```python
from build123d import *

# Parameters (mm, degrees)
F0_R     = 5.25
F1_DEPTH = 12
F2_DEPTH = 11
F3_DEPTH = 12
F4_SIZE  = 1
F5_SIZE  = 1


with BuildPart() as f1:
    # F0 (on Top) → F1 (new body)
    with BuildSketch(Plane.XY):
        with BuildLine():
            ThreePointArc((4, -17.036725), (13.715867, -10.868533), (17.5, 0))
            ThreePointArc((17.5, 0), (-10.868533, 13.715867), (-4, -17.036725))
            ThreePointArc((-4, -17.036725), (0, -17.5), (4, -17.036725))
        make_face()
        Circle(F0_R, mode=Mode.SUBTRACT)
        Circle(F0_R)
        with BuildLine():
            ThreePointArc((2.727178, 1.25), (2.931001, 0.639713), (3, 0))
            ThreePointArc((3, 0), (-0.639713, -2.931001), (-2.727178, 1.25))
            ThreePointArc((-2.727178, 1.25), (0, 3), (2.727178, 1.25))
        make_face(mode=Mode.SUBTRACT)
        with BuildLine():
            ThreePointArc((-2.727178, 1.25), (-0.639713, -2.931001), (3, 0))
            ThreePointArc((3, 0), (2.931001, 0.639713), (2.727178, 1.25))
            Line((2.727178, 1.25), (-2.727178, 1.25))
        make_face()
        with BuildLine():
            Line((-2.727178, 1.25), (2.727178, 1.25))
            ThreePointArc((2.727178, 1.25), (0, 3), (-2.727178, 1.25))
        make_face()
    extrude(amount=F1_DEPTH)

    # F0 (on Top) → F2 (join)
    with BuildSketch(Plane.XY):
        Circle(F0_R)
        with BuildLine():
            ThreePointArc((2.727178, 1.25), (2.931001, 0.639713), (3, 0))
            ThreePointArc((3, 0), (-0.639713, -2.931001), (-2.727178, 1.25))
            ThreePointArc((-2.727178, 1.25), (0, 3), (2.727178, 1.25))
        make_face(mode=Mode.SUBTRACT)
        with BuildLine():
            Line((-2.727178, 1.25), (2.727178, 1.25))
            ThreePointArc((2.727178, 1.25), (0, 3), (-2.727178, 1.25))
        make_face()
    extrude(amount=-F2_DEPTH)

    # F0 (on Top) → F3 (join)
    with BuildSketch(Plane.XY):
        with BuildLine():
            ThreePointArc((4, -17.036725), (0, -17.5), (-4, -17.036725))
            Line((-4, -17.036725), (0, -22.5))
            Line((0, -22.5), (4, -17.036725))
        make_face()
    extrude(amount=F3_DEPTH)

    # F4
    f4_edges = [f1.edges().sort_by_distance(p)[0] for p in [
        (0, 17.5, 0),
        (-2, -19.768363, 0),
        (2, -19.768363, 0),
        (-5.25, 0, 0),
    ]]
    chamfer(f4_edges, length=F4_SIZE)

    # F5
    f5_edges = [f1.edges().sort_by_distance(p)[0] for p in [
        (0, 17.5, 12),
        (-2, -19.768363, 12),
        (2, -19.768363, 12),
    ]]
    chamfer(f5_edges, length=F5_SIZE)


solid = f1.part
```
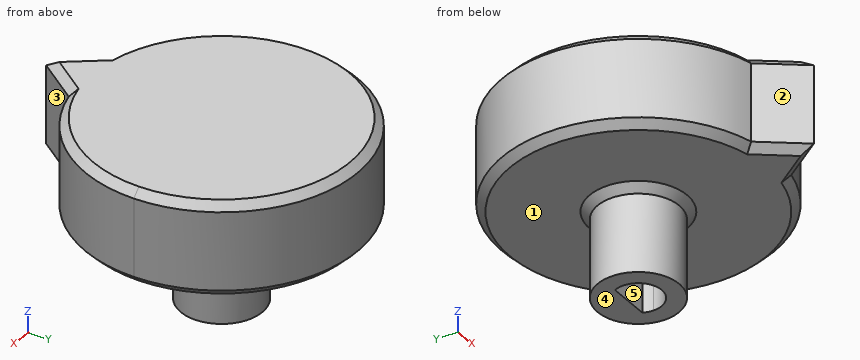
Design review of the part built by this model. Coordinates are the model's own, in mm. Face numbers are marked on the shaded views. A direction names the side the tool comes from. Give positions to 0.01 mm unless a question says otherwise; leave off trailing zeros. Order: outer loops, then holes, each group sorted by start corner. A loop starts at its lowest first (then second) coordinate and runs counter-clockwise, first axis right, second up. Notation, with made-up numbers: M 70,64.5 L 107,64.5 A20 cw 107,82.5 Z; hole C -4.75,-25 d1. An arc over 180 degrees is marked long. One line per question, with ' | ' between items. Start each with the question number.
Q1. We need section C-C (z = 10.5). Write out the cut boundary in (x, y).
Q2. For L1, parallel to Y at x = 0, z = -3.75; L2, parallel to Z at x = 3, y = 7; L3, parallel to Y at x = -2, z = -1, list the stretches that pass through material, from the lowest coordinate up. Write a range as [from, to].
Q3. The part is to be moulded in two halves that separate along Y. For the marked faces 3, 4 and 5, say which applies: +Y half, -Y half, draft (parallel to the pull), parting line (faces both ways), or undercut.
Q4. We need section B-B (y = -18.5). Write out the cut boundary in (x, z).
Q5. For pin 1 Ø3.5 at (x, y) = (0, 0) entering from -Z; pin 2 Ø1.6 at (x, z) = (0, -6) entering from -Y; pin 3 Ø2 at (x, z) = (-2.5, -4) entering from +Y; pin 4 Ø10 at (y, z) = (4, -8) entering from -X, all flat-tipped, find the tip position at first contact; note any pin that passes through.
Q6. Machinability: for the marked faces 1 and 2, which of the approach directions +Z, -Z, +X, -X, +Y, -Y give a long, thin tool a straight path to every point of the face, cutting with its end or side? Answer none if there is none.
Q7. We need section A-A (z = -4.5). Write out the cut boundary in (x, y), plus the area to 3 significant figures.
Returned:
1) outline: M -4,-17.04 L 0,-22.5 L 4,-17.04 A17.5 ccw 17.5,0 A17.5 ccw long Z
2) L1: [-5.25, -3], [1.25, 5.25] | L2: [0, 12] | L3: [-4.85, -2.24], [1.25, 4.85]
3) face 3: -Y half | face 4: draft | face 5: undercut
4) outline: M -2.93,1 L -1.69,0 L 1.69,0 L 2.93,1 L 2.93,11 L 1.69,12 L -1.69,12 L -2.93,11 Z
5) pin 1: z = -11 | pin 2: y = -5.25 | pin 3: y = 5.03 | pin 4: x = -5.25
6) face 1: -Z | face 2: +Z, -Z, -X, -Y
7) outline: C 0,0 d10.5; hole M -2.73,1.25 A3 ccw long 3,0 A3 ccw 2.73,1.25 Z | area: 65.2 mm2
